Could you check a few things on this model? Use its own coordinates, in mm. A direction names the side the tool comes from. Give positions to 0.01 mm unless a question says otherwise; leave off trailing zeros. Write each loop counter-clockwise with the first axis right and the second up, starting at its lowest first coordinate (ties: lowest second). Pieces come first, ordered by that corner, then holes. Notation, with made-up numbers: (63, 17.5) -> (69, 17.5) arc R16 cw to (69, 44.5) -> close; hole circle Ø6 at (70, 27.25). An arc over 180 degrees is marked (long way). One line per question, with ' | ' between items.
from build123d import *

# Parameters (mm, degrees)
BOSS_EXTRUDE1_DEPTH = 2.54
CHAMFER1_SIZE       = 3.81
CUT_EXTRUDE1_DEPTH  = 124.039639744
CUT_EXTRUDE2_DEPTH  = 124.039639744
FILLET1_R           = 1.27


with BuildPart() as part:
    # Sketch1 → Boss-Extrude1 (new body)
    with BuildSketch(Plane.XY):
        Polygon((5.842, 0), (16.2941, 0), (16.2941, 33.782), (98.8441, 33.782), (98.8441, 0), (109.2962, 0), (109.2962, 2.794), (115.1382, 2.794), (115.1382, 33.782), (109.2962, 33.782), (109.2962, 43.307), (5.842, 43.307), (5.842, 33.782), (0, 33.782), (0, 2.794), (5.842, 2.794), align=None)
    extrude(amount=BOSS_EXTRUDE1_DEPTH)

    # Chamfer1
    chamfer1_edges = [part.edges().sort_by_distance(p)[0] for p in [
        (5.842, 43.307, 1.27),
        (109.2962, 43.307, 1.27),
    ]]
    chamfer(chamfer1_edges, length=CHAMFER1_SIZE)

    # Sketch2 → Cut-Extrude1 (cut, through all)
    with BuildSketch(Plane.XY.offset(2.54)):
        Polygon((0, 33.782), (5.842, 33.782), (5.842, 17.995192435), (16.2941, 17.995192435), (16.2941, -3.098792672), (0, -3.098792672), align=None)
    extrude(amount=-CUT_EXTRUDE1_DEPTH, mode=Mode.SUBTRACT)

    # Sketch3 → Cut-Extrude2 (cut, through all)
    with BuildSketch(Plane.XY.offset(2.54)):
        Polygon((109.2962, 33.782), (115.1382, 33.782), (115.1382, -2.224430595), (98.8441, 0), (42.867468811, 17.995192435), (109.2962, 17.995192435), align=None)
    extrude(amount=-CUT_EXTRUDE2_DEPTH, mode=Mode.SUBTRACT)

    # Fillet1
    fillet1_edges = [part.edges().sort_by_distance(p)[0] for p in [
        (16.2941, 17.995192435, 1.27),
        (5.842, 17.995192435, 1.27),
        (98.8441, 17.995192435, 1.27),
        (109.2962, 17.995192435, 1.27),
    ]]
    fillet(fillet1_edges, radius=FILLET1_R)


solid = part.part
Q1. Will this pin go through, and if not, where does the flat tip stop? pin 1 (1.3 mm diameter, centred on x = 57, z = 1, fed in from -Y).
Answer below:
pin 1: stops at y = 33.78
Q2. Imagine slicing it at B-B on z = 0.5. Please give me the cut outline in (x, y).
Answer below:
outline: (5.84, 19.27) arc R1.27 ccw to (7.11, 18) -> (15.02, 18) arc R1.27 ccw to (16.29, 19.27) -> (16.29, 33.78) -> (98.84, 33.78) -> (98.84, 19.27) arc R1.27 ccw to (100.11, 18) -> (108.03, 18) arc R1.27 ccw to (109.3, 19.27) -> (109.3, 39.5) -> (105.49, 43.31) -> (9.65, 43.31) -> (5.84, 39.5) -> close
Q3. Imagine slicing it at C-C on x = 24.5. Please give me the cut outline in (y, z), and give its area (3 significant figures).
Answer below:
outline: (33.78, 0) -> (43.31, 0) -> (43.31, 2.54) -> (33.78, 2.54) -> close | area: 24.2 mm^2
Q4. If we mould it in two halves opening along X, with no side actions, what happens to faces 3 (the flat face through (16.294, 26, 1)), 4 (the flat face through (5.842, 30, 1)), 5 (the flat face through (57, 36, 2.54))? For each: +X half, -X half, draft (parallel to the pull), parting line (faces both ways), or undercut.
Answer below:
face 3: undercut | face 4: -X half | face 5: draft
Q5. Imagine slicing it at A-A on y = 21.25. Please give me the cut outline in (x, z), and give its area (3 significant figures).
Answer below:
outline: (5.84, 0) -> (16.29, 0) -> (16.29, 2.54) -> (5.84, 2.54) -> close; (98.84, 0) -> (109.3, 0) -> (109.3, 2.54) -> (98.84, 2.54) -> close | area: 53.1 mm^2
Q6. On a 3-axis mill with a long thin cutter (end or side, diameter ignored), from which of +Z, -Z, +X, -X, +Y, -Y can I reach the whole of each face in a straight line? I mean faces 1 (the flat face through (98.844, 27, 1)), 2 (the flat face through (11, 17.995, 1)). Say none if no direction works.
Answer below:
face 1: +Z, -Z, -Y | face 2: +Z, -Z, +X, -X, -Y
Q7. If I drill on line 1 along X through (y, z) = (32.5, 2.35); line 2 along Y through (x, z) = (17, 0.8); line 3 along X through (y, z) = (40, 2) (3 decimals), over which ranges is the centre line in solid material (lowest first)?
Answer below:
line 1: x = 5.84 to 16.29, 98.84 to 109.3 | line 2: y = 33.78 to 43.31 | line 3: x = 6.345 to 108.793
